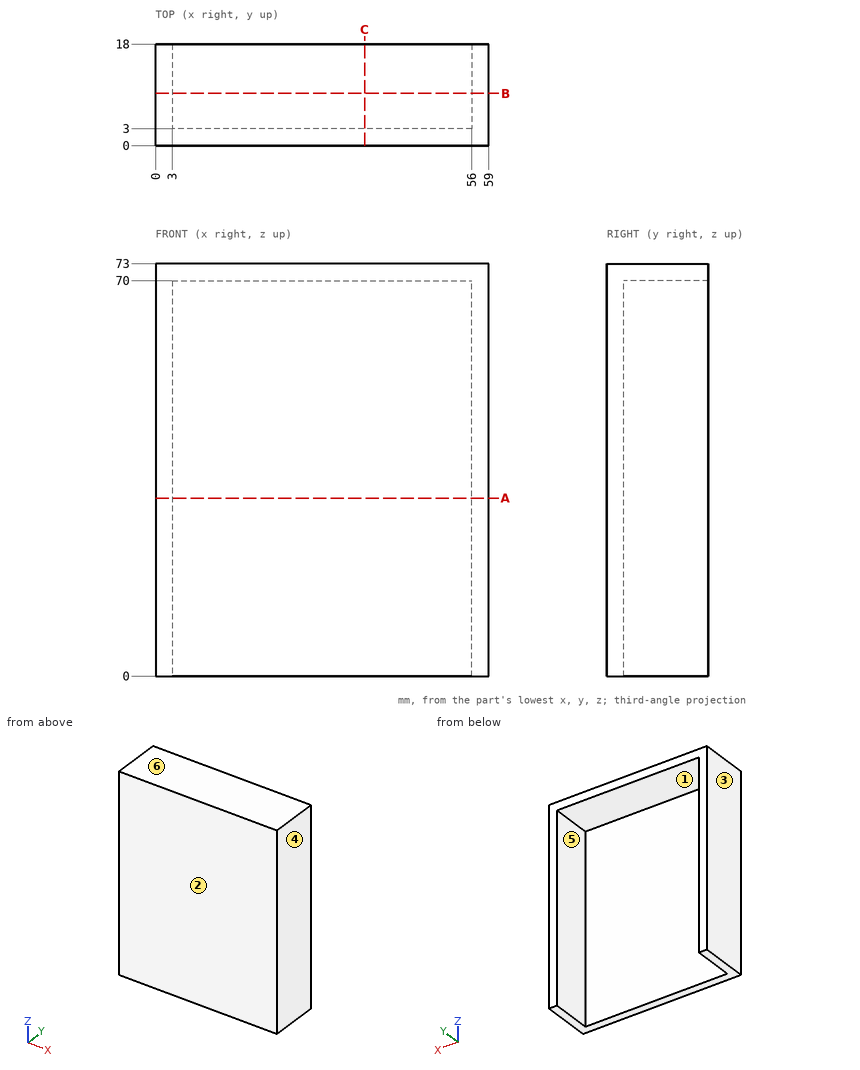
Source: three-view drawing plus pictorial views. Frame: mm from the lowest corner of the part. A direction names the side the tool comes from. Round coordinates to 2 decimals unless told otherwise and drop trailing zeros. Write each loop counter-clockwise with the first axis right and the second up, starting at its lowest first coordinate (ties: lowest second). Pieces come first, ordered by that corner, then holes. Notation, with made-up numbers: M 27,39 L 44,39 A28 cw 44,74 Z; hole C 48.5,62.5 d9. An arc over 180 degrees is marked long. Use CSV: the item, a comma, the result in double quotes. Start each with the question number.
Q1. Pull-direction query (X, two-part tool) for the marked faces 1, 2, 3 and 4; classes: +X half, -X half, draft (parallel to the pull), parting line (faces both ways), or undercut.
Q2. Access query for the marked faces 5 and 6. Directions: +Z, -Z, +X, -X, +Y, -Y. A direction counts if a zero-diameter tool reaches every point of the face in a straight line with its end or side. Return the directions, or none.
Q3. Cut plane A-A on z = 31.5. Output: boundary loops of the cut face in (x, y).
Q4. Cut plane C-C on x = 37. Output: boundary loops of the cut face in (y, z).
Q5. First-contact query: P1, Ø6, axis at x = 11, y = 3, coming from the -Z side; P2, Ø10, axis at x = 19.5, z = 60.5, coming from the +Y side; P3, Ø4.5, axis at x = 16.5, y = 7, coming from the -Z side. Flat tips, straight axial feed; report the tip coordinate or a pass-through.
Q6. Line query: line 1 (X direction, y = 11.5, z = 60); line 2 (Z direction, x = 17.5, y = 14.75); line 3 (Y direction, x = 45, z = 35). Output: solid intervals per line, ascending. Write a range as from..to.
Q7. Cut plane B-B on y = 9.25. Output: boundary loops of the cut face in (x, z), plus the area to 3 significant figures.
Results found:
1,face 1,"undercut"
1,face 2,"draft"
1,face 3,"-X half"
1,face 4,"+X half"
2,face 5,"-Z, +Y"
2,face 6,"+Z, +X, -X, +Y, -Y"
3,outline,"M 0,0 L 59,0 L 59,18 L 56,18 L 56,3 L 3,3 L 3,18 L 0,18 Z"
4,outline,"M 0,0 L 3,0 L 3,70 L 18,70 L 18,73 L 0,73 Z"
5,P1,"z = 0"
5,P2,"y = 3"
5,P3,"z = 70"
6,line 1,"0..3, 56..59"
6,line 2,"70..73"
6,line 3,"0..3"
7,outline,"M 0,0 L 3,0 L 3,70 L 56,70 L 56,0 L 59,0 L 59,73 L 0,73 Z"
7,area,"597 mm^2"
